from build123d import *

# Parameters (mm, degrees)
ESBO_O1_W                = 48
ESBO_O1_H                = 35
ESBO_O1_R                = 2.5
RESSALTO_EXTRUS_O1_DEPTH = 2
ESBO_O2_W                = 4
ESBO_O2_H                = 35
RESSALTO_EXTRUS_O2_DEPTH = 38
ESBO_O3_W                = 48
ESBO_O3_H                = 21.220088249
ESBO_O3_R                = 5
RESSALTO_EXTRUS_O3_DEPTH = 2


with BuildPart() as part:
    # Esboço1 → Ressalto-extrusão1 (new body)
    with BuildSketch(Plane.XY):
        with Locations((-27.792174024, -21.17139219)):
            Rectangle(ESBO_O1_W, ESBO_O1_H)
        with Locations((-27.810949966, -21.337629256)):
            Circle(ESBO_O1_R, mode=Mode.SUBTRACT)
    extrude(amount=RESSALTO_EXTRUS_O1_DEPTH)

    # Esboço2 → Ressalto-extrusão2 (add)
    with BuildSketch(Plane.XY.offset(2)):
        with Locations((-49.792174024, -21.17139219)):
            Rectangle(ESBO_O2_W, ESBO_O2_H)
        with Locations((-5.792174024, -21.17139219)):
            Rectangle(ESBO_O2_W, ESBO_O2_H)
    extrude(amount=RESSALTO_EXTRUS_O2_DEPTH)

    # Esboço3 → Ressalto-extrusão3 (add)
    with BuildSketch(Plane.XZ.offset(38.67139219)):
        with Locations((-27.792174024, 29.389955876)):
            Rectangle(ESBO_O3_W, ESBO_O3_H)
        with Locations(Location((-39.792174024, 29.389955876, 0), (0, 0, 270))):
            Circle(ESBO_O3_R, mode=Mode.SUBTRACT)
        with Locations(Location((-15.792174024, 29.389955876, 0), (0, 0, 270))):
            Circle(ESBO_O3_R, mode=Mode.SUBTRACT)
    extrude(amount=RESSALTO_EXTRUS_O3_DEPTH)


solid = part.part
The listing builds one solid part. Answer for the finished solid, in the listing's coordinates (mm). A direction names the side the tool comes from. Give positions to 0.01 mm unless a question says otherwise; leave off trailing zeros. Write each loop counter-clockwise with the first axis right and the second up, starting at its lowest first coordinate (ties: lowest second). Pieces come first, ordered by that corner, then holes.
Item 1: Section A-A, the plane z = 18 is taken. Write down the section's boundary in (x, y).
Item 2: Determine the mould class of faces 1 (the flat face through (-27.9, -38.671, 1.7)), 2 (the flat face through (-51.792, -22, 20)), 3 (the cylindrical face through (-44.673, -39.657, 30.474)), 4 (the flat face through (-3.792, -22, 20)) for opening direction X: released by +X, released by -X, zero draft, split by the parting line, or undercut.
Item 3: Section D-D, the plane x = -12.5 is taken. Write down the section's boundary in (y, z).
Item 4: Section C-C, the plane z = 27 is taken. Write down the section's boundary in (x, y), plus the area to 3 significant figures.
Item 5: Find the intervals of material crossed by line 1 along X through (y, z) = (-33, 10.5); line 2 along Z through (x, y) = (-44.5, -33); line 3 along Y through (x, z) = (-46, 30), in increasing order.
Item 6: Flat-ended cylindrical pins translate along their axes: P1, Ø3, axis at x = -41, y = -34.5, coming from the +Z side; P2, Ø20.5, axis at x = -32.5, z = 7, coming from the -Y side; P3, Ø6, axis at x = -39.79, z = 29.39, coming from the +Y side; P4, Ø6.5, axis at x = -25, z = 25.5, coming from the +Y side. Find the tip coordinate at first contact, or state that the pin passes through.
Item 7: Which of the six approach directions +Z, -Z, +X, -X, +Y, -Y give full straight-line access (tool end or side, diameter ignored) to faces 5 (the flat face through (-28, -40.671, 30)), 6 (the flat face through (-28, -40, 40)), 7 (the flat face through (-28, -40, 18.78)), 8 (the flat face through (-47.792, -21, 21)), 9 (the flat face through (-28, -17, 2))?
Item 8: Section B-B, the plane x = -31 is taken. Write down the section's boundary in (y, z).
Completed:
1. outline: (-51.79, -38.67) - (-47.79, -38.67) - (-47.79, -3.67) - (-51.79, -3.67) - close; (-7.79, -38.67) - (-3.79, -38.67) - (-3.79, -3.67) - (-7.79, -3.67) - close
2. face 1: zero draft
2. face 2: released by -X
2. face 3: undercut
2. face 4: released by +X
3. outline: (-40.67, 18.78) - (-38.67, 18.78) - (-38.67, 25.63) - (-40.67, 25.63) - close; (-40.67, 33.15) - (-38.67, 33.15) - (-38.67, 40) - (-40.67, 40) - close; (-38.67, 0) - (-3.67, 0) - (-3.67, 2) - (-38.67, 2) - close
4. outline: (-51.79, -40.67) - (-44.18, -40.67) - (-44.18, -38.67) - (-47.79, -38.67) - (-47.79, -3.67) - (-51.79, -3.67) - close; (-35.4, -40.67) - (-20.18, -40.67) - (-20.18, -38.67) - (-35.4, -38.67) - close; (-11.4, -40.67) - (-3.79, -40.67) - (-3.79, -3.67) - (-7.79, -3.67) - (-7.79, -38.67) - (-11.4, -38.67) - close
4. area: 341 mm2
5. line 1: x = -51.79 to -47.79, -7.79 to -3.79
5. line 2: z = 0 to 2
5. line 3: y = -40.67 to -38.67
6. P1: stops at z = 2
6. P2: stops at y = -38.67
6. P3: passes through
6. P4: stops at y = -38.67
7. face 5: +Z, -Z, +X, -X, -Y
7. face 6: +Z, +X, -X, +Y, -Y
7. face 7: -Z, +X, -X, -Y
7. face 8: +Z, +Y
7. face 9: +Z, +Y, -Y
8. outline: (-40.67, 18.78) - (-38.67, 18.78) - (-38.67, 40) - (-40.67, 40) - close; (-38.67, 0) - (-3.67, 0) - (-3.67, 2) - (-38.67, 2) - close
